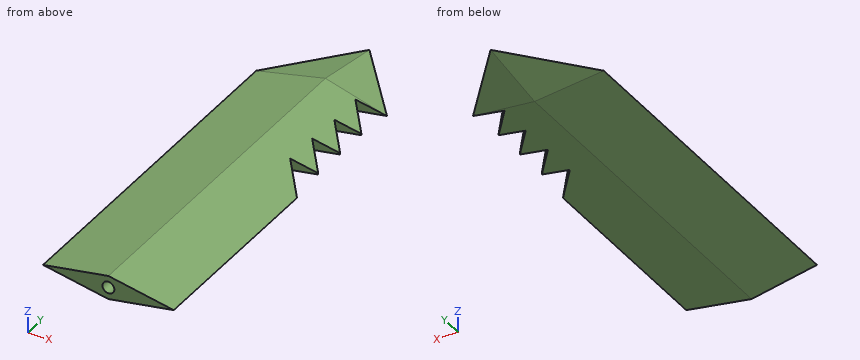
```python
from build123d import *

# Parameters (mm, degrees)
BOSS_EXTRUDE1_DEPTH      = 9.525
BOSS_EXTRUDE1_DEPTH_BACK = 9.525
CUT_EXTRUDE1_DEPTH       = 373.680910299
CUT_EXTRUDE2_DEPTH       = 373.680910299
SKETCH5_W                = 97.518379051
SKETCH5_H                = 136.419580789
CUT_EXTRUDE3_DEPTH       = 739.741184154
SKETCH6_W                = 75.100700845
SKETCH6_H                = 154.277977479
CUT_EXTRUDE4_DEPTH       = 748.678846608
SKETCH7_R                = 4.7625
CUT_EXTRUDE5_DEPTH       = 254


with BuildPart() as part:
    # Sketch1 → Boss-Extrude1 (new, two sides: drawn at the far end of the back side and taken through both)
    with BuildSketch(Plane.XY.offset(-BOSS_EXTRUDE1_DEPTH_BACK)):
        Polygon((101.792411443, 735.656458749), (49.404911443, 673.557276224), (49.404911443, 396.497366015), (154.179911443, 396.497366015), (154.179911443, 556.636391043), (128.683999881, 589.063224066), (151.148766449, 589.063224066), (128.683999881, 617.634912224), (151.148766449, 617.634912224), (129.452026088, 645.229790529), (151.148766449, 645.229790529), (128.876006433, 673.557276224), (154.179911443, 673.557276224), align=None)
    extrude(amount=BOSS_EXTRUDE1_DEPTH + BOSS_EXTRUDE1_DEPTH_BACK)

    # Sketch2 → Cut-Extrude1 (cut, through all)
    with BuildSketch(Plane(origin=(0, 396.497366015, 0), x_dir=(-1, 0, 0), z_dir=(0, -1, 0))):
        Polygon((-49.404911443, 0), (-101.792411443, -9.525), (-154.179911443, 0), (-159.65732669, 0), (-159.65732669, -13.649148588), (-44.158493861, -13.649148588), (-44.158493861, 0), align=None)
    extrude(amount=-CUT_EXTRUDE1_DEPTH, mode=Mode.SUBTRACT)

    # Sketch3 → Cut-Extrude2 (cut, through all)
    with BuildSketch(Plane.XZ.offset(-396.497366015)):
        Polygon((49.404911443, 0), (101.792411443, -9.525), (154.179911443, 0), (159.580570647, 0), (159.580570647, -14.500746269), (43.682013433, -14.500746269), (43.682013433, 0), align=None)
    extrude(amount=-CUT_EXTRUDE2_DEPTH, mode=Mode.SUBTRACT)

    # Sketch5 → Cut-Extrude3 (cut, through all)
    with BuildSketch(Plane(origin=(26.430459561, 22.297003663, 133.782021979), x_dir=(0.9815360247212257, -0.031445805879602766, -0.1886748352776165), z_dir=(0.1912773697394791, 0.16136352846789567, 0.9681811708073739))):
        with Locations((89.248369642, 700.742830845)):
            Rectangle(SKETCH5_W, SKETCH5_H)
    cut_extrude3 = extrude(amount=CUT_EXTRUDE3_DEPTH, mode=Mode.SUBTRACT)

    # Sketch6 → Cut-Extrude4 (cut, through all)
    with BuildSketch(Plane(origin=(-18.981895096, 16.01331916, 96.079914958), x_dir=(0.9815360247212258, 0.03144580587960229, 0.18867483527761636), z_dir=(-0.19127736973947887, 0.1613635284678934, 0.9681811708073744))):
        with Locations((98.873573013, 697.792784398)):
            Rectangle(SKETCH6_W, SKETCH6_H)
    cut_extrude4 = extrude(amount=CUT_EXTRUDE4_DEPTH, mode=Mode.SUBTRACT)

    # Mirror1: Cut-Extrude3, Cut-Extrude4 across plane
    add(cut_extrude3.mirror(Plane.XY), mode=Mode.SUBTRACT)
    add(cut_extrude4.mirror(Plane.XY), mode=Mode.SUBTRACT)

    # Sketch7 → Cut-Extrude5 (cut)
    with BuildSketch(Plane.XZ.offset(-396.497366015)):
        with Locations(Location((101.792411443, 0, 0), (0, 0, 270))):
            Circle(SKETCH7_R)
    extrude(amount=-CUT_EXTRUDE5_DEPTH, mode=Mode.SUBTRACT)


solid = part.part
```
Geometry check sheet. Reference: the model listing, model coordinates, mm. Round coordinates to 2 decimals unless told otherwise and drop trailing zeros. Loops run counter-clockwise (first coordinate to the right, second up) from the corner with the lowest first, then second, coordinate; pieces in that order, holes last. Notation, with made-up numbers: M 41,86 L 66,86 A27 cw 66,107 Z; hole C -7.5,-9.75 d5. An arc over 180 degrees is marked long. Return JSON: item names as keys, results as strings. Group by question number.
(1) Section check C-C, the plane x = 57. Enter the section's corners in (y, z).
(2) Go/stop test with flat-tipped pins: pin 1 (8 mm diameter, centred on y = 552.5, z = -1.5, fed in from +X); pin 2 (1 mm diameter, centred on x = 92, y = 701, fed in from +Z); pin 3 (3 mm diameter, centred on x = 102.5, z = -1, fed in from -Y). Record where each tip stops, or that it passes through.
(3) Section check A-A, the plane y = 490.5. Enter the section's corners in (x, z) (1 decimal).
(4) Scan lines: line 1 along Z through (x, y) = (75.5, 540.5); line 2 along Z through (x, y) = (103, 552); line 3 along Z through (x, y) = (116.5, 446). Record each from-to range of solid material in increasing order. Write a range as [from, to].
(5) Section check B-B, the plane x = 112.5. Enter the section's corners in (y, z), and give its area (3 significant figures).
Data:
{
 "1": {"outline": "M 396.5,-1.38 L 674.27,-1.38 L 682.56,0 L 674.27,1.38 L 396.5,1.38 Z"},
 "2": {"pin 1": "x = 154.18", "pin 2": "z = 3.97", "pin 3": "y = 650.5"},
 "3": {"outline": "M 49.4,0 L 101.8,-9.5 L 154.2,0 L 101.8,9.5 Z; hole C 101.8,0 d9.5"},
 "4": {"line 1": "[-4.74, 4.74]", "line 2": "[-9.31, -4.61], [4.61, 9.31]", "line 3": "[-6.85, 6.85]"},
 "5": {"outline": "M 396.5,-7.58 L 677.49,-7.58 L 722.96,0 L 677.49,7.58 L 396.5,7.58 Z", "area": "4,600 mm²"}
}
